Design review of the part built by this model. Coordinates are the model's own, in mm. Face numbers are marked on the shaded views. Round coordinates to 2 decimals unless told otherwise and drop trailing zeros. Order: outer loops, then holes, each group sorted by start corner. A loop starts at its lowest first (then second) coordinate and runs counter-clockwise, first axis right, second up. Notation, with made-up numbers: (48, -29) - (72, -29) arc R15 cw to (72, -11) - close; hole circle Ø3 at (-38, 41). An arc over 180 degrees is marked (long way). Write item = value, one per line.
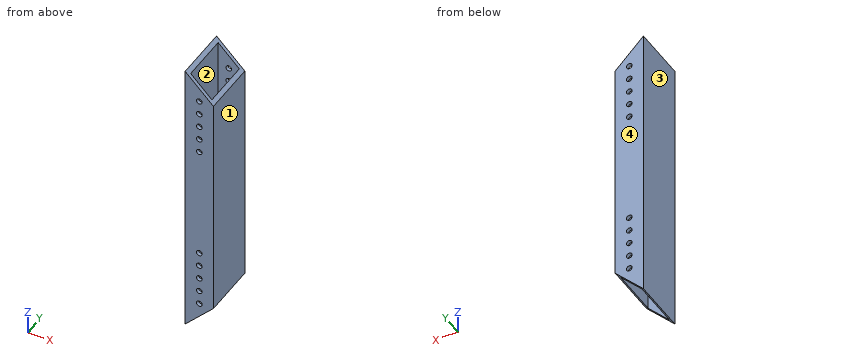
Autodesk Inventor part; units mm, degrees
ref_plane "YZ Plane" through (0, 0, 0) normal (1, 0, 0) x (0, 1, 0)
ref_plane "XZ Plane" through (0, 0, 0) normal (0, 1, 0) x (-1, 0, 0)
ref_plane "XY Plane" through (0, 0, 0) normal (0, 0, 1) x (1, 0, 0)
sketch "Sketch1" plane through (0, 0, 0) normal (0, 0, 1) x (1, 0, 0)
  line L0 (-12.7, -25.4) -> (12.7, -25.4)
  line L1 (12.7, -25.4) -> (12.7, 25.4)
  line L2 (12.7, 25.4) -> (-12.7, 25.4)
  line L3 (-12.7, 25.4) -> (-12.7, -25.4)
  line L4 (-12.7, -25.4) -> (12.7, 25.4) construction
  line L5 (12.7, -25.4) -> (-12.7, 25.4) construction
  line L6 (-9.525, 22.225) -> (9.525, 22.225)
  line L7 (9.525, 22.225) -> (9.525, -22.225)
  line L8 (9.525, -22.225) -> (-9.525, -22.225)
  line L9 (-9.525, -22.225) -> (-9.525, 22.225)
  point P0 (0, 0)
  dimension "d0" = 25.4
  dimension "d1" = 50.8
  dimension "d2" = 3.175
extrude "Extrusion1" add sketch "Sketch1" along normal mid plane 254
sketch "Sketch2" plane through (-12.7, -25.4, 127) normal (0, -1, 0) x (1, 0, 0)
  line L0 (25.4, 0) -> (25.4, -254)
  line L1 (0, 0) -> (25.4, 0) construction
  line L2 (0, -254) -> (0, 0) construction
  line L3 (25.4, -254) -> (0, -254)
  line L4 (0, -254) -> (25.4, -228.6)
  point P0 (12.7, -127)
  dimension "d6" = 45
extrude "Extrusion2" cut sketch "Sketch2" against normal through all
sketch "Sketch4" plane through (-12.7, -25.4, 127) normal (0, -1, 0) x (1, 0, 0)
  line L0 (0, -254) -> (0, 0) construction
  point P0 (12.7, -127)
  point P1 (12.7, -228.6)
  point P2 (12.7, -215.9)
  point P3 (12.7, -203.2)
  point P4 (12.7, -190.5)
  point P5 (12.7, -177.8)
  dimension "d9" = 12.7
  dimension "d10" = 25.4
  dimension "d13" = 12.7
hole "Hole1" at (0, -25.4, -101.6) at (0, -25.4, -88.9) at (0, -25.4, -76.2) at (0, -25.4, -63.5) at (0, -25.4, -50.8) direction (0, 1, 0) diameter 5.1054 end through all
mirror "Mirror1" about plane through (0, 0, 0) normal (0, 0, 1) of "Hole1", "Extrusion2"
properties part number "TUBE,ELEVATOR,BOT,STAGE1" material "Aluminum 6061 T6 0 Cold Formed"
1) The part is to be moulded in two halves that separate along X. For the marked faces 1, 2, 3 and 4, say which applies: released by +X, released by -X, zero draft, split by the parting line, or undercut.
Findings:
face_1 = released by +X
face_2 = undercut
face_3 = released by -X
face_4 = zero draft
2) To check wall thickness, follow L1, parallel to X at y = 23, z = 63; L2, parallel to Y at x = -2.5, z = -92 (3 decimals); L3, parallel to X at y = 5.5, z = -51 (3 decimals). State the ranges of each line that lie inside material, in increasing order. Write a range as from..to.
Findings:
L1 = -12.7..-2.5, 2.5..12.7
L2 = -25.4..-22.225, 22.225..25.4
L3 = -12.7..-9.525, 9.525..12.7
3) We need section B-B on z = -76.2. Write out the cut boundary in (x, y) (3 decimals), and give its area (3 significant figures).
Findings:
outline = (-12.7, -25.4) - (-2.553, -25.4) - (-2.553, -22.225) - (-9.525, -22.225) - (-9.525, 22.225) - (-2.553, 22.225) - (-2.553, 25.4) - (-12.7, 25.4) - close; (2.553, -25.4) - (12.7, -25.4) - (12.7, 25.4) - (2.553, 25.4) - (2.553, 22.225) - (9.525, 22.225) - (9.525, -22.225) - (2.553, -22.225) - close
area = 411 mm^2
4) We need section A-A on y = -11. Write out the cut boundary in (x, z) (3 decimals), and give its area (3 significant figures).
Findings:
outline = (-12.7, -127) - (-9.525, -123.825) - (-9.525, 123.825) - (-12.7, 127) - close; (9.525, -104.775) - (12.7, -101.6) - (12.7, 101.6) - (9.525, 104.775) - close
area = 1,450 mm^2
5) We need section C-C on x = 0. Give the number of separate pieces and of enclosed holes in the cut face, and give its area (3 significant figures).
Findings:
separate_pieces = 22
enclosed_holes = 0
area = 1,130 mm^2
